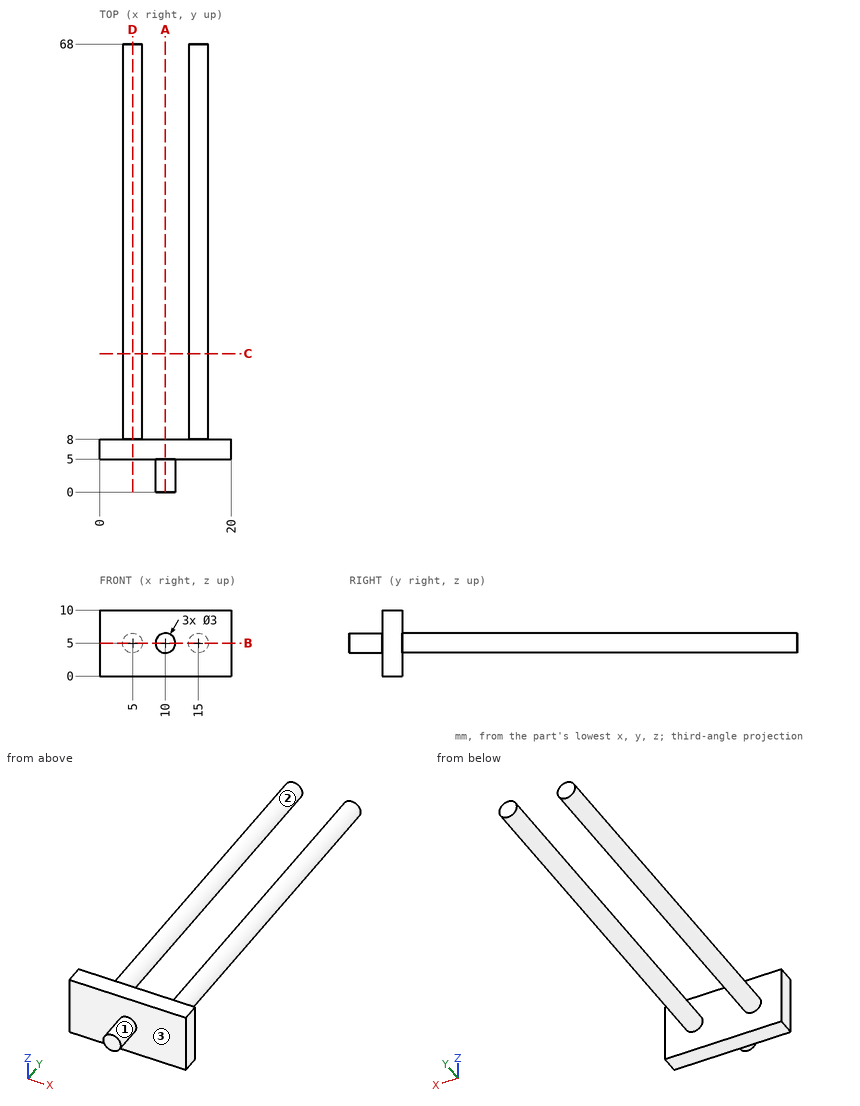
Here's the drawing with two shaded views (mm, measured from the low corner). I have some questions. Coordinates: 2 decimals unless noted, no trailing zeros. Loops run counter-clockwise (first coordinate to the right, second up) from the corner with the lowest first, then second, coordinate; pieces in that order, holes last. Notation, with made-up numbers: (1.25, 7.25) -> (6.25, 7.25) arc R19 cw to (6.25, 12.25) -> close; hole circle Ø2 at (89, -38.5). An arc over 180 degrees is marked (long way). Use one line per item in the form item = value. Start each with the question number.
(1) If we section it at B-B (z = 5): Please give me the cut outline in (x, y).
(2) If we section it at A-A (x = 10): Please give me the cut outline in (y, z), then the cut area to 3 significant figures.
(3) Will these pins go through, and if not, where does the flat tip stop? pin 1 (4 mm diameter, centred on y = 57, z = 6, fed in from -X); pin 2 (2 mm diameter, centred on x = 5, z = 4.5, fed in from -Y); pin 3 (4 mm diameter, centred on y = 57.5, z = 3.5, fed in from +X); pin 4 (12 mm diameter, centred on x = 16, y = 9, fed in from +Z).
(4) We'd pull the mould along X, two halves only. Please class the marked faces 1, 2 and 3: pulls with the +X half, pulls with the -X half, needs draft (parallel to the pull), parting line crosses it, or undercut.
(5) If we section it at D-D (x = 5): Please give me the cut outline in (y, z).
(6) Please list where these lines run through material, in increasing order: line 1 along Y through (x, z) = (11.25, 4.75); line 2 along Y through (x, z) = (7.25, 3.75); line 3 along X through (y, z) = (37, 5.75).
(7) If we section it at C-C (y = 21): Please give me the cut outline in (x, z).
Verdict:
q1.outline = (0, 5) -> (8.5, 5) -> (8.5, 0) -> (11.5, 0) -> (11.5, 5) -> (20, 5) -> (20, 8) -> (16.5, 8) -> (16.5, 68) -> (13.5, 68) -> (13.5, 8) -> (6.5, 8) -> (6.5, 68) -> (3.5, 68) -> (3.5, 8) -> (0, 8) -> close
q2.outline = (0, 3.5) -> (5, 3.5) -> (5, 0) -> (8, 0) -> (8, 10) -> (5, 10) -> (5, 6.5) -> (0, 6.5) -> close
q2.area = 45.0 mm²
q3.pin_1 = 3.5
q3.pin_2 = 5
q3.pin_3 = 16.5
q3.pin_4 = 10
q4.face_1 = parting line crosses it
q4.face_2 = undercut
q4.face_3 = needs draft
q5.outline = (5, 0) -> (8, 0) -> (8, 3.5) -> (68, 3.5) -> (68, 6.5) -> (8, 6.5) -> (8, 10) -> (5, 10) -> close
q6.line_1 = 0 to 8
q6.line_2 = 5 to 8
q6.line_3 = 3.7 to 6.3, 13.7 to 16.3
q7.outline = circle Ø3 at (5, 5); circle Ø3 at (15, 5)
